Verification items for the finished model (mm, model axes). A direction names the side the tool comes from. Coordinates: 2 decimals unless noted, no trailing zeros. Order: outer loops, then holes, each group sorted by start corner. A loop starts at its lowest first (then second) coordinate and runs counter-clockwise, first axis right, second up. Notation, with made-up numbers: M -5.5,32.5 L 12.5,32.5 A21 ccw 12.5,66.5 Z; hole C -17.75,40 d8. An arc over 180 degrees is marked long. Return JSON: item names as keys, results as strings. Group by question number.
Q1. Section check B-B, the plane x = 0. Enter the section's corners in (y, z) (3 decimals).
Q2. Section check A-A, the plane z = 0. Enter the section's corners in (x, y) (3 decimals), then the cut area to 3 significant figures.
Q3. Section check C-C, the plane z = 15.5. Enter the section's corners in (x, y) (3 decimals), then the cut area to 3 significant figures.
Q4. Go/stop test with a flat-tipped pin: pin 1 Ø1.5 at (x, y) = (10.5, 1.5) entering from +Z. Record where the tip stops, or that it passes through.
Q5. Thickness scan on probe 1 along Z at (x, y) = (15.5, 2.3) (3 decimals); probe 2 along Z at (x, y) = (21.5, 2.45) (3 decimals). Record the ranges inside material, lowest first.
Q6. Mould release check, pull along X, two halves, no side actions. Record for faces 1 (the face through (-23, 2, -9.5)), 2 (the face through (24.325, 2, 19)), 3 (the face through (13.5, 2, 23)): pulls with the +X half, pulls with the -X half, needs draft (parallel to the pull), parting line crosses it, or undercut.
Q7. Access from +Z, -Z, +X, -X, +Y, -Y to the whole of each face (thin tool, end or side, straight path). Record for faces 4 (the face through (-9.5, 2, -23)), 5 (the face through (-12, 2, 21.15)), 6 (the face through (23, 2, 2)), 7 (the face through (-23, 2, 9.5)), 8 (the face through (-16.64, 1.57, -16.55)).
Q8. Section check D-D, the plane x = 15.5. Enter the section's corners in (y, z) (3 decimals), then the cut area to 3 significant figures.
from build123d import *

# Parameters (mm, degrees)
SKETCH2_R           = 1.55
SKETCH2_R_2         = 11
BOSS_EXTRUDE1_DEPTH = 3.175


with BuildPart() as part:
    # Sketch2 → Boss-Extrude1 (new body)
    with BuildSketch(Plane(origin=(0, 0, 0), x_dir=(1, 0, 0), z_dir=(0, 1, 0))):
        Polygon((24.325, 2), (24.325, 9.5), (21.15, 9.5), (21.15, 13.5), (24.325, 13.5), (24.325, 24.325), (13.5, 24.325), (13.5, 21.15), (9.5, 21.15), (9.5, 24.325), (2, 24.325), (2, 21.15), (-2, 21.15), (-2, 24.325), (-9.5, 24.325), (-9.5, 21.15), (-13.5, 21.15), (-13.5, 24.325), (-24.325, 24.325), (-24.325, 13.5), (-21.15, 13.5), (-21.15, 9.5), (-24.325, 9.5), (-24.325, 2), (-21.15, 2), (-21.15, -2), (-24.325, -2), (-24.325, -9.5), (-21.15, -9.5), (-21.15, -13.5), (-24.325, -13.5), (-24.325, -24.325), (-13.5, -24.325), (-13.5, -21.15), (-9.5, -21.15), (-9.5, -24.325), (-2, -24.325), (-2, -21.15), (2, -21.15), (2, -24.325), (9.5, -24.325), (9.5, -21.15), (13.5, -21.15), (13.5, -24.325), (24.325, -24.325), (24.325, -13.5), (21.15, -13.5), (21.15, -9.5), (24.325, -9.5), (24.325, -2), (21.15, -2), (21.15, 2), align=None)
        with Locations((-15.5, -15.5)):
            Circle(SKETCH2_R, mode=Mode.SUBTRACT)
        with Locations((15.5, -15.5)):
            Circle(SKETCH2_R, mode=Mode.SUBTRACT)
        Circle(SKETCH2_R_2, mode=Mode.SUBTRACT)
        with Locations((-15.5, 15.5)):
            Circle(SKETCH2_R, mode=Mode.SUBTRACT)
        with Locations((15.5, 15.5)):
            Circle(SKETCH2_R, mode=Mode.SUBTRACT)
    extrude(amount=BOSS_EXTRUDE1_DEPTH)


solid = part.part
Numbers:
{
 "1": {"outline": "M 0,-21.15 L 3.175,-21.15 L 3.175,-11 L 0,-11 Z; M 0,11 L 3.175,11 L 3.175,21.15 L 0,21.15 Z"},
 "2": {"outline": "M -21.15,0 L -11,0 L -11,3.175 L -21.15,3.175 Z; M 11,0 L 21.15,0 L 21.15,3.175 L 11,3.175 Z", "area": "64.5 mm2"},
 "3": {"outline": "M -24.325,0 L -17.05,0 L -17.05,3.175 L -24.325,3.175 Z; M -13.95,0 L 13.95,0 L 13.95,3.175 L -13.95,3.175 Z; M 17.05,0 L 24.325,0 L 24.325,3.175 L 17.05,3.175 Z", "area": "135 mm2"},
 "4": {"pin 1": "stops at z = 21.15"},
 "5": {"probe 1": "z = -24.325 to -17.05, -13.95 to 13.95, 17.05 to 24.325", "probe 2": "z = -24.325 to -13.5, -9.5 to -2, 2 to 9.5, 13.5 to 24.325"},
 "6": {"face 1": "needs draft", "face 2": "pulls with the +X half", "face 3": "undercut"},
 "7": {"face 4": "-Z, +Y, -Y", "face 5": "+Z, +Y, -Y", "face 6": "+X, +Y, -Y", "face 7": "-X, +Y, -Y", "face 8": "+Y, -Y"},
 "8": {"outline": "M 0,-24.325 L 3.175,-24.325 L 3.175,-17.05 L 0,-17.05 Z; M 0,-13.95 L 3.175,-13.95 L 3.175,13.95 L 0,13.95 Z; M 0,17.05 L 3.175,17.05 L 3.175,24.325 L 0,24.325 Z", "area": "135 mm2"}
}
